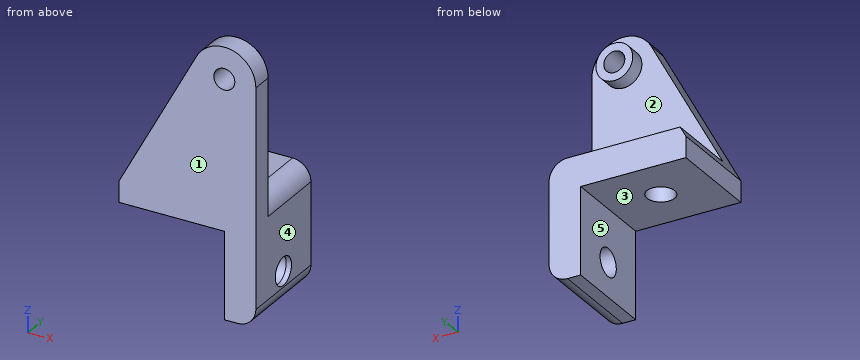
```python
from build123d import *

# Parameters (mm, degrees)
PAD013_DEPTH         = 9
POCKET017_DEPTH      = 14.001
SKETCH042_R          = 3.5
PAD014_DEPTH         = 3
SKETCH044_R          = 2
POCKET018_DEPTH      = 4.001
POCKET018_DEPTH_BACK = 14.001
SKETCH045_R          = 2.65
POCKET019_DEPTH      = 34.351
POCKET019_DEPTH_BACK = 16.501
SKETCH046_R          = 2.65
POCKET020_DEPTH      = 25.001
POCKET020_DEPTH_BACK = 1.001


with BuildPart() as part:
    # Sketch041 → Pad013 (new body, symmetric)
    with BuildSketch(Plane(origin=(0, 0, 0), x_dir=(-1, 0, 0), z_dir=(0, 1, 0))):
        with BuildLine():
            Line((-26, 28.35), (-26, -13))
            ThreePointArc((-26, -13), (-24.974874, -15.474874), (-22.5, -16.5))
            Line((-22.5, -16.5), (-20, -16.5))
            Line((-20, -16.5), (-20, 0))
            Line((-20, 0), (0, 0))
            Line((0, 0), (0, 4))
            Line((0, 4), (-14.723172, 31.205711))
            ThreePointArc((-14.723172, 31.205711), (-21.472928, 34.166398), (-26, 28.35))
        make_face()
    extrude(amount=PAD013_DEPTH, both=True)

    # Sketch043 → Pocket017 (cut, through all)
    with BuildSketch(Plane(origin=(0, -5, 0), x_dir=(-1, 0, 0), z_dir=(0, 1, 0))):
        with BuildLine():
            Line((-26, 2.5), (-26, 40))
            Line((-26, 40), (0, 40))
            Line((0, 40), (0, 6))
            Line((0, 6), (-22.5, 6))
            ThreePointArc((-22.5, 6), (-24.974874, 4.974874), (-26, 2.5))
        make_face()
    extrude(amount=POCKET017_DEPTH, mode=Mode.SUBTRACT)

    # Sketch042 → Pad014 (join)
    with BuildSketch(Plane(origin=(0, -5, 0), x_dir=(-1, 0, 0), z_dir=(0, 1, 0))):
        with Locations((-20, 28.35)):
            Circle(SKETCH042_R)
    extrude(amount=PAD014_DEPTH)

    # Sketch044 → Pocket018 (cut, two sides)
    with BuildSketch(Plane(origin=(0, -5, 0), x_dir=(-1, 0, 0), z_dir=(0, 1, 0))) as pocket018_sk:
        with Locations((-20, 28.35)):
            Circle(SKETCH044_R)
    extrude(amount=-POCKET018_DEPTH, mode=Mode.SUBTRACT)
    extrude(pocket018_sk.sketch, amount=POCKET018_DEPTH_BACK, mode=Mode.SUBTRACT)

    # Sketch045 → Pocket019 (cut, two sides)
    with BuildSketch(Plane(origin=(10, 0, 0), x_dir=(1, 0, 0), z_dir=(0, 0, 1))) as pocket019_sk:
        Circle(SKETCH045_R)
    extrude(amount=POCKET019_DEPTH, mode=Mode.SUBTRACT)
    extrude(pocket019_sk.sketch, amount=-POCKET019_DEPTH_BACK, mode=Mode.SUBTRACT)

    # Sketch046 → Pocket020 (cut, two sides)
    with BuildSketch(Plane(origin=(25, 0, -10), x_dir=(0, 1, 0), z_dir=(1, 0, 0))) as pocket020_sk:
        Circle(SKETCH046_R)
    extrude(amount=-POCKET020_DEPTH, mode=Mode.SUBTRACT)
    extrude(pocket020_sk.sketch, amount=POCKET020_DEPTH_BACK, mode=Mode.SUBTRACT)


with BuildPart() as part_1:
    # Body018 placement: moved
    add(part.part.moved(Location((0, 39, 0))))


solid = part_1.part
```
Geometry check sheet. Reference: the model listing, model coordinates, mm. Face numbers are marked on the shaded views. A direction names the side the tool comes from. Give positions to 0.01 mm unless a question says otherwise; leave off trailing zeros. Order: outer loops, then holes, each group sorted by start corner. A loop starts at its lowest first (then second) coordinate and runs counter-clockwise, first axis right, second up. Notation, with made-up numbers: (-9.75, -20) -> (42.25, -20) arc R8 ccw to (42.25, -9) -> close; hole circle Ø1 at (-36.75, -22). An arc over 180 degrees is marked (long way). Write each question's results on one line, items separated by ' | '. Start each with the question number.
(1) Mould release check, pull along Z, two halves, no side actions. Record for the marked faces 1, 2 and 3: pulls with the +Z half, pulls with the -Z half, needs draft (parallel to the pull), parting line crosses it, or undercut.
(2) Sectioned sample at B-B (z = -10). Enter the section's corners in (x, y).
(3) Sectioned sample at C-C (x = 21.25). Enter the section's corners in (y, z), plus the area to 3 significant figures.
(4) Gauge pin test, flat ends, axial feed: P1, Ø3.5, axis at x = 18.5, z = 28.5, coming from the +Y side; P2, Ø10, axis at y = 43.5, z = -4.5, coming from the -X side; P3, Ø1.5, axis at y = 32, z = 12, coming from the -X side; P4, Ø6, axis at x = 6.5, y = 40.5, coming from the +Z side. Record the tip position at first contact, or that the pin passes through.
(5) Sectioned sample at A-A (y = 35.5). Enter the section's corners in (x, z), plus the area to 3 significant figures.
(6) Scan lines: line 1 (Y direction, x = 25.6, z = -10); line 2 (Y direction, x = 18, z = 26.5); line 3 (Y direction, x = 8.75, z = 8.5). Record each from-to range of solid material in increasing order.
(7) Access from +Z, -Z, +X, -X, +Y, -Y to the whole of each face (thin tool, end or side, straight path). Record for the marked faces 4 and 5.
(8) Sectioned sample at D-D (x = 10). Enter the section's corners in (y, z).
Answer below:
1) face 1: needs draft | face 2: undercut | face 3: pulls with the -Z half
2) outline: (20, 30) -> (26, 30) -> (26, 36.35) -> (20, 36.35) -> close; (20, 41.65) -> (26, 41.65) -> (26, 48) -> (20, 48) -> close
3) outline: (30, -16.5) -> (48, -16.5) -> (48, 6) -> (34, 6) -> (34, 25.08) -> (37, 25.08) -> (37, 26.79) -> (30, 26.79) -> close; (30, 29.91) -> (37, 29.91) -> (37, 31.62) -> (34, 31.62) -> (34, 34.22) -> (30, 34.22) -> close; hole circle Ø5.3 at (39, -10) | area: 494 mm2
4) P1: y = 37 | P2: x = 0 | P3: x = 3.92 | P4: z = 6
5) outline: (0, 0) -> (20, 0) -> (20, -16.5) -> (22.5, -16.5) arc R3.5 ccw to (26, -13) -> (26, 2.5) arc R3.5 ccw to (22.5, 6) -> (1.08, 6) -> (0, 4) -> close; circle Ø7 at (20, 28.35); hole circle Ø4 at (20, 28.35) | area: 275 mm2
6) line 1: 30 to 36.35, 41.65 to 48 | line 2: 30 to 37 | line 3: 30 to 34
7) face 4: +Z, -Z, +X, +Y, -Y | face 5: -Z, -X, +Y, -Y
8) outline: (30, 0) -> (36.35, 0) -> (36.35, 6) -> (34, 6) -> (34, 22.48) -> (30, 22.48) -> close; (41.65, 0) -> (48, 0) -> (48, 6) -> (41.65, 6) -> close
